Can you work these out from the model? Positions are in its coordinate system, mm. Give positions to 0.01 mm unless a question says otherwise; leave off trailing zeros. Loops run counter-clockwise (first coordinate to the right, second up) from the corner with the lowest first, then second, coordinate; pieces in that order, holes last. Notation, with made-up numbers: (43, 52.5) -> (80, 52.5) arc R15 ccw to (80, 62.5) -> close; hole circle Ø4 at (18, 23). An arc over 180 degrees is marked (long way). Return JSON: item names as keys, results as strings. Group by question number.
Q1. I need wall thicknesses on line 1 along Y through (x, z) = (32.5, 5.5); line 2 along Y through (x, z) = (9.5, 6); line 3 along X through (y, z) = (58, -26). Which ranges of each line are inside material? Lowest first, please. Write a range as [from, to].
Q2. Suppose I cut it at A-A, the plane x = -9.5. Please give me the cut outline in (y, z).
Q3. Will these pins go through, and if not, where does the flat tip stop? pin 1 (4 mm diameter, centred on y = 53, z = -18.5, fed in from -X); pin 2 (5 mm diameter, centred on x = 26, z = -4, fed in from -Y); pin 3 (1 mm diameter, centred on x = 26, y = 88, fed in from -Z); pin 4 (10 mm diameter, centred on x = -8, y = 55, fed in from -Z).
Q4. Suppose I cut it at B-B, the plane z = 0. Please give me the cut outline in (x, y), and give its area (3 significant figures).
Q5. Suppose I cut it at C-C, the plane y = 76. Please give me the cut outline in (x, z), and give its area (3 significant figures).
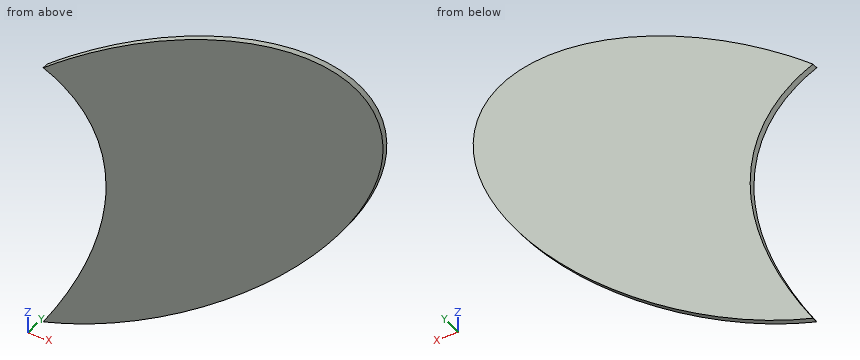
```python
from build123d import *

# Parameters (mm, degrees)
SKETCH4_W               = 232.52141371
SKETCH4_H               = 186.000175814
BOSS_EXTRUDE1_DEPTH     = 1
SKETCH1_OUTSIDE_W       = 226.832
SKETCH1_OUTSIDE_H       = 247.708
SKETCH1_OUTSIDE_R       = 35.5
CUT_EXTRUDE2_DEPTH      = 185.225637078
CUT_EXTRUDE3_DEPTH      = 109.319901238
CUT_EXTRUDE3_DEPTH_BACK = 109.319901238
SKETCH5_R               = 62.5


with BuildPart() as part:
    # Sketch4 → Boss-Extrude1 (new body)
    with BuildSketch(Plane(origin=(-30.241408096, 30.241408096, 0), x_dir=(0.7071067811865512, 0.7071067811865439, 0), z_dir=(0.7071067811865439, -0.7071067811865512, 0))):
        Rectangle(SKETCH4_W, SKETCH4_H)
    extrude(amount=BOSS_EXTRUDE1_DEPTH)

    # Sketch1 outside → Cut-Extrude2 (cut, through all)
    with BuildSketch(Plane(origin=(0, 0, 0), x_dir=(1, 0, 0), z_dir=(0, 1, 0))):
        with Locations((-29.888, 0)):
            Rectangle(SKETCH1_OUTSIDE_W, SKETCH1_OUTSIDE_H)
        with Locations(Location((0, 0, 0), (0, 0, 180))):
            Circle(SKETCH1_OUTSIDE_R, mode=Mode.SUBTRACT)
    extrude(amount=CUT_EXTRUDE2_DEPTH, mode=Mode.SUBTRACT)


with BuildPart() as body_2:
    # of the pieces the cut leaves, the one that is kept (cut_extrude2_keep)
    add(part.part.solids().sort_by_distance((-35.5, 24.982816193, 0))[0])

    # Sketch5 → Cut-Extrude3 (cut, two sides: drawn at the far end of the back side and taken through both)
    with BuildSketch(Plane(origin=(0, 0, 0), x_dir=(1, 0, 0), z_dir=(0, 1, 0)).offset(-CUT_EXTRUDE3_DEPTH_BACK)):
        with Locations((-67.416033427, 0)):
            Circle(SKETCH5_R)
    extrude(amount=CUT_EXTRUDE3_DEPTH + CUT_EXTRUDE3_DEPTH_BACK, mode=Mode.SUBTRACT)


solid = body_2.part
```
Ans:
{
 "1": {"line 1": "y = [91.57, 92.98]", "line 2": "y = [68.57, 69.98]", "line 3": "x = [-2.48, -1.07]"},
 "2": {"outline": "(49.57, -34.21) -> (50.98, -34.21) -> (50.98, -23.49) -> (49.57, -23.49) -> close; (49.57, 23.49) -> (50.98, 23.49) -> (50.98, 34.21) -> (49.57, 34.21) -> close"},
 "3": {"pin 1": "stops at x = -8.31", "pin 2": "stops at y = 82.57", "pin 3": "passes through", "pin 4": "stops at z = -35.36"},
 "4": {"outline": "(-4.92, 54.15) -> (35.5, 94.57) -> (35.5, 95.98) -> (-4.92, 55.57) -> close", "area": "57.2 mm^2"},
 "5": {"outline": "(15.52, -31.93) arc R35.5 ccw to (16.93, -31.2) -> (16.93, 31.2) arc R35.5 ccw to (15.52, 31.93) -> close", "area": "89.3 mm^2"}
}
